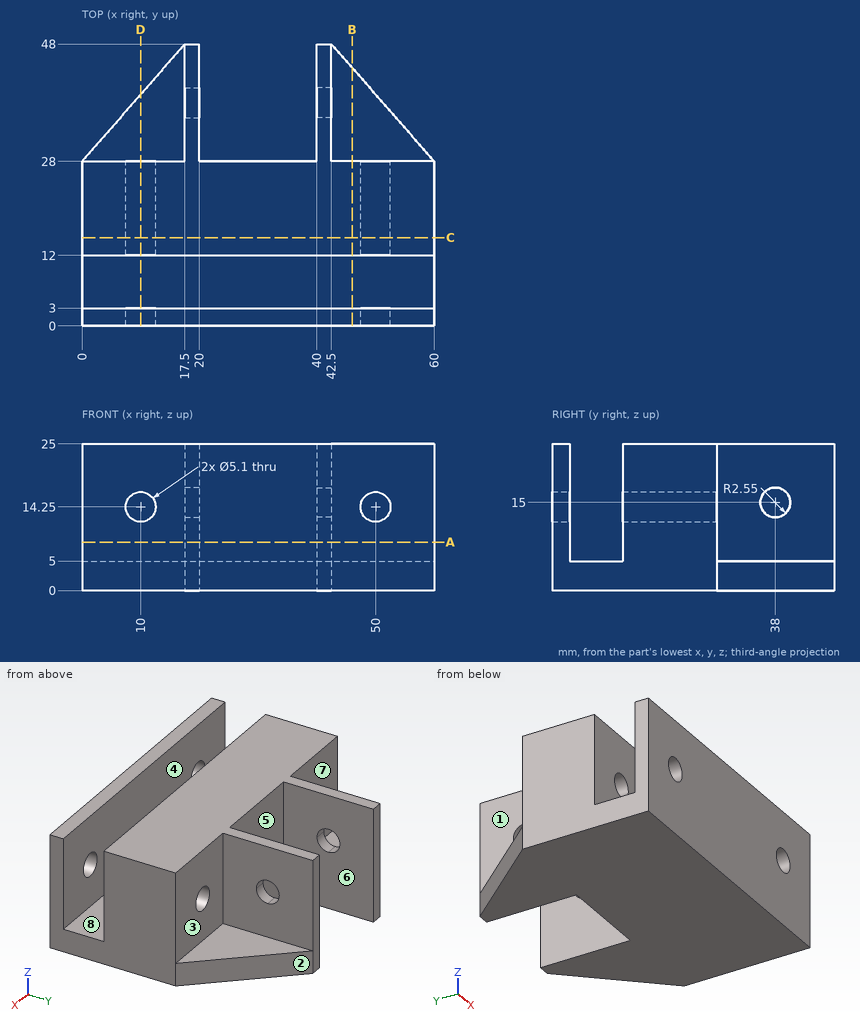
Study the drawing (mm; zero at the part's minimum x, y, z) and answer. A direction names the side the tool comes from. Coordinates: 2 decimals unless noted, no trailing zeros. Write each loop counter-clockwise with the first axis right and the second up, starting at its lowest first coordinate (ties: lowest second). Pieces come first, ordered by that corner, then holes. Notation, with made-up numbers: M 8,67.5 L 27,67.5 A12 cw 27,90.5 Z; hole C 33,-19.5 d6. An arc over 180 degrees is marked long. Use a Markdown table: item, result. Add a question column.
1. Section B-B (x = 46) is taken. Give the vertices of the cut face in (y, z).
2. For a pull along Y with two mould halves and no side action, classify the marked faces 6, 7 and 8 as +Y half, -Y half, draft (parallel to the pull), parting line (faces both ways), or undercut.
3. Which of the six approach directions +Z, -Z, +X, -X, +Y, -Y give full straight-line access (tool end or side, diameter ignored) to the marked faces 1, 2, 3, 4 and 5?
4. Straight lines are drawn through the part: line 1 along X through (y, z) = (40.5, 23.75); line 2 along Y through (x, z) = (23, 15.5); line 3 along X through (y, z) = (1.9, 14.25). For each, find the intervals that lie inside material, in ascending order. Write a range as [from, to].
5. Section A-A (z = 8.25) is taken. Give the vertices of the cut face in (x, y).
6. Given P1, Ø1, axis at y = 30, z = 13, coming from the +X side; P2, Ø6.5, axis at x = 50, z = 14.25, coming from the +Y side; P3, Ø4.5, axis at x = 10, z = 14.25, coming from the +Y side; P4, Ø5, axis at x = 48, y = 38.5, coming from the +Z side, each flat-ended and moving along its own axis, determine where each tip first touches the part or whether it passes through.
7. Section D-D (x = 10) is taken. Give the vertices of the cut face in (y, z).
8. Section C-C (y = 15) is taken. Give the vertices of the cut face in (x, z).
Data:
| question | item | result |
|---|---|---|
| 1 | outline | M 0,0 L 44,0 L 44,5 L 28,5 L 28,25 L 12,25 L 12,5 L 3,5 L 3,25 L 0,25 Z |
| 2 | face 6 | draft |
| 2 | face 7 | +Y half |
| 2 | face 8 | undercut |
| 3 | face 1 | +Z, -X, +Y |
| 3 | face 2 | +Z, -Z, +X, +Y |
| 3 | face 3 | +Z, +X, +Y |
| 3 | face 4 | +Z, +X, -X |
| 3 | face 5 | +Z, -Z, +Y |
| 4 | line 1 | x = [17.5, 20], [40, 42.5] |
| 4 | line 2 | y = [0, 3], [12, 28] |
| 4 | line 3 | x = [0, 7.45], [12.55, 47.45], [52.55, 60] |
| 5 | outline | M 0,0 L 60,0 L 60,3 L 0,3 Z; M 0,12 L 60,12 L 60,28 L 42.5,28 L 42.5,48 L 40,48 L 40,28 L 20,28 L 20,48 L 17.5,48 L 17.5,28 L 0,28 Z |
| 6 | P1 | stops at x = 42.5 |
| 6 | P2 | stops at y = 28 |
| 6 | P3 | passes through |
| 6 | P4 | stops at z = 5 |
| 7 | outline | M 0,0 L 39.43,0 L 39.43,5 L 28,5 L 28,11.7 L 12,11.7 L 12,5 L 3,5 L 3,11.7 L 0,11.7 Z; M 0,16.8 L 3,16.8 L 3,25 L 0,25 Z; M 12,16.8 L 28,16.8 L 28,25 L 12,25 Z |
| 8 | outline | M 0,0 L 60,0 L 60,25 L 0,25 Z; hole C 10,14.25 d5.1; hole C 50,14.25 d5.1 |
